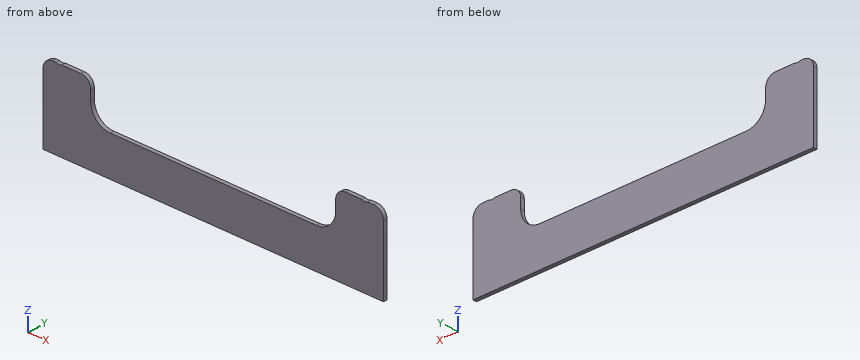
from build123d import *

# Parameters (mm, degrees)
EXTRUDE_1_DEPTH          = 6
CUT_EXTRUDE_1_DEPTH      = 14
CUT_EXTRUDE_1_DEPTH_BACK = 5
SKETCH_7_R               = 11
CUT_EXTRUDE_2_DEPTH      = 11
CUT_EXTRUDE_2_DEPTH_BACK = 5
SKETCH_8_R               = 11


with BuildPart() as part:
    # Эскиз1 → Бобышка-Вытянуть1 (new body)
    with BuildSketch(Plane(origin=(0, 0, 0), x_dir=(1, 0, 0), z_dir=(0, 1, 0))):
        with BuildLine():
            Line((-338.202898551, 15), (-338.202898551, 120))
            Line((-338.202898551, 120), (189.797101449, 120))
            Line((189.797101449, 120), (189.797101449, 15))
            ThreePointArc((189.797101449, 15), (185.403703167, 4.393398282), (174.797101449, 0))
            Line((174.797101449, 0), (130.797101449, 0))
            ThreePointArc((130.797101449, 0), (120.190499731, 4.393398282), (115.797101449, 15))
            Line((115.797101449, 15), (115.797101449, 30))
            ThreePointArc((115.797101449, 30), (107.010304885, 51.213203436), (85.797101449, 60))
            Line((85.797101449, 60), (-234.202898551, 60))
            ThreePointArc((-234.202898551, 60), (-255.416101986, 51.213203436), (-264.202898551, 30))
            Line((-264.202898551, 30), (-264.202898551, 15))
            ThreePointArc((-264.202898551, 15), (-268.596296833, 4.393398282), (-279.202898551, 0))
            Line((-279.202898551, 0), (-323.202898551, 0))
            ThreePointArc((-323.202898551, 0), (-333.809500269, 4.393398282), (-338.202898551, 15))
        make_face()
    extrude(amount=EXTRUDE_1_DEPTH)

    # Эскиз7 → Вырез-Вытянуть1 (cut, two sides: drawn at the far end of the back side and taken through both)
    with BuildSketch(Plane(origin=(0, 0, 0), x_dir=(1, 0, 0), z_dir=(0, 1, 0)).offset(-CUT_EXTRUDE_1_DEPTH_BACK)):
        with Locations((-313.202898551, -10)):
            Circle(SKETCH_7_R)
    extrude(amount=CUT_EXTRUDE_1_DEPTH + CUT_EXTRUDE_1_DEPTH_BACK, mode=Mode.SUBTRACT)

    # Эскиз8 → Вырез-Вытянуть2 (cut, two sides: drawn at the far end of the back side and taken through both)
    with BuildSketch(Plane(origin=(0, 0, 0), x_dir=(1, 0, 0), z_dir=(0, 1, 0)).offset(-CUT_EXTRUDE_2_DEPTH_BACK)):
        with Locations((160.797101449, -10)):
            Circle(SKETCH_8_R)
    extrude(amount=CUT_EXTRUDE_2_DEPTH + CUT_EXTRUDE_2_DEPTH_BACK, mode=Mode.SUBTRACT)


solid = part.part
The model under review builds one solid part; all positions refer to its coordinate system, in mm. Coordinates: 2 decimals unless noted, no trailing zeros. Write each loop counter-clockwise with the first axis right and the second up, starting at its lowest first coordinate (ties: lowest second). Pieces come first, ordered by that corner, then holes. Notation, with made-up numbers: (24.5, -17.75) - (52.5, -17.75) arc R22 ccw to (52.5, 7.25) - close; hole circle Ø9 at (41.25, -19.5). An arc over 180 degrees is marked (long way). Answer as CSV lines item,"result".
(1) For line 1 along X through (y, z) = (3.75, -23); line 2 along Z through (x, y) = (-116, 3.85); line 3 along X through (y, z) = (0.6, -40), list the stretches that pass through material, from the lowest coordinate up. Write a range as [from, to].
Data:
line 1,"x = [-338.2, -264.2], [115.8, 189.8]"
line 2,"z = [-120, -60]"
line 3,"x = [-338.2, -262.49], [114.08, 189.8]"
(2) We need section C-C (x = 58). Give the boundary of the cut face in (y, z), plus the area to 3 significant figures.
Data:
outline,"(0, -120) - (6, -120) - (6, -60) - (0, -60) - close"
area,"360 mm2"
(3) We need section D-D (z = -50.5). Give the boundary of the cut face in (x, y).
Data:
outline,"(-338.2, 0) - (-256.11, 0) - (-256.11, 6) - (-338.2, 6) - close; (107.7, 0) - (189.8, 0) - (189.8, 6) - (107.7, 6) - close"
(4) Clearance check with flat-ended pins moving along their axes: pin 1 Ø1.8 at (x, y) = (-18, 4.5) entering from +Z; pin 2 Ø3 at (y, z) = (3.5, -12) entering from +X; pin 3 Ø3 at (x, y) = (-274, 5) entering from +Z. State where each tip first meets the part, or that it passes through.
Data:
pin 1,"stops at z = -60"
pin 2,"stops at x = 189.72"
pin 3,"stops at z = -0.46"
(5) We need section A-A (z = -25.5). Give the boundary of the cut face in (x, y), plus the area to 3 significant figures.
Data:
outline,"(-338.2, 0) - (-264.2, 0) - (-264.2, 6) - (-338.2, 6) - close; (115.8, 0) - (189.8, 0) - (189.8, 6) - (115.8, 6) - close"
area,"888 mm2"
(6) We need section B-B (y = 5.05). Give the boundary of the cut face in (x, z).
Data:
outline,"(-338.2, -120) - (189.8, -120) - (189.8, -15) arc R15 ccw to (174.8, 0) - (165.38, 0) arc R11 cw to (156.21, 0) - (130.8, 0) arc R15 ccw to (115.8, -15) - (115.8, -30) arc R30 cw to (85.8, -60) - (-234.2, -60) arc R30 cw to (-264.2, -30) - (-264.2, -15) arc R15 ccw to (-279.2, 0) - (-308.62, 0) arc R11 cw to (-317.79, 0) - (-323.2, 0) arc R15 ccw to (-338.2, -15) - close"
